Here's how the part is built. I have some questions about the finished solid (model axes, mm). A direction names the side the tool comes from. Round coordinates to 2 decimals unless told otherwise and drop trailing zeros. Write each loop counter-clockwise with the first axis right and the second up, starting at its lowest first coordinate (ties: lowest second). Pieces come first, ordered by that corner, then holes. Notation, with made-up numbers: M 62,15 L 80,15 A29 ccw 80,49 Z; hole C -16.75,-24.5 d11. An arc over 180 degrees is marked long. Write item = value, one per line. Start each with the question number.
(1) I need wall thicknesses on line 1 along Y through (x, z) = (35.5, 18.75); line 2 along Y through (x, z) = (-15.5, 4); line 3 along X through (y, z) = (-6.5, 10.5). Which ranges of each line are inside material? Lowest first, please.
(2) On a 3-axis mill with a long thin cutter (end or side, diameter ignored), from which of +Z, -Z, +X, -X, +Y, -Y can I reach the whole of each face in a straight line? I mean faces 5 (the flat face through (-0.367, 23.785, 22.535)), 6 (the flat face through (80, -35, 6)). Say none if no direction works.
(3) Will these pins go through, and if not, where does the flat tip stop? pin 1 Ø7.5 at (y, z) = (-9, 15.5) entering from -X; pin 2 Ø7.5 at (y, z) = (13.5, 10) entering from +X; pin 3 Ø2 at (x, z) = (64, 6) entering from +Y.
(4) I want a section at A-A (z = 3.5). Give the number of separate pieces and of enclosed holes in the cut face, and give its area (3 significant figures).
(5) I want a section at B-B (x = -15.5). List the corners of the cut face in (y, z) for me, and give its area (3 significant figures).
(6) If we mould it in two halves opening along X, with no side actions, what happens to faces 1 (the flat face through (-21.25, 0, 15)), 2 (the flat face through (65, -30, 12)), 3 (the cylindrical face through (51, -28, 13)), 4 (the cylindrical face through (13.9, 15.57, 4.93))? For each: released by +X, released by -X, zero draft, split by the parting line, or undercut.
(7) I want a section at D-D (y = 0). List the corners of the cut face in (x, z) for me.
(8) I want a section at C-C (y = -15.5). List the corners of the cut face in (x, z) for me.
```python
from build123d import *

# Parameters (mm, degrees)
F0_R      = 4.1
F0_W      = 42.5
F0_H      = 42.5
F0_W_2    = 30
F0_H_2    = 10
F1_DEPTH  = 25
F0_R_2    = 1.6
F0_R_3    = 6
F2_DEPTH  = 10
F3_SIZE   = 5
F4_R      = 5
F5_R      = 5
F6_R      = 2.1
F7_DEPTH  = 25
F8_R      = 12.5
F9_R      = 2.1
F10_DEPTH = 25


with BuildPart() as f1:
    # F0 (on Top) → F1 (new body)
    with BuildSketch(Plane.XY):
        Polygon((-50, -30), (-50, -40), (50, -40), (50, -30), (50, 40), (-50, 40), align=None)
        with Locations((-35.5, -30.5)):
            Circle(F0_R, mode=Mode.SUBTRACT)
        with Locations((35.5, -30.5)):
            Circle(F0_R, mode=Mode.SUBTRACT)
        with Locations((-35.5, 30.5)):
            Circle(F0_R, mode=Mode.SUBTRACT)
        Rectangle(F0_W, F0_H, mode=Mode.SUBTRACT)
        with Locations((35.5, 30.5)):
            Circle(F0_R, mode=Mode.SUBTRACT)
        with Locations((-65, -35)):
            Rectangle(F0_W_2, F0_H_2)
        with Locations((65, -35)):
            Rectangle(F0_W_2, F0_H_2)
    extrude(amount=F1_DEPTH)

    # F0 (on Top) → F2 (join)
    with BuildSketch(Plane.XY):
        Rectangle(F0_W, F0_H)
        with Locations((-15.5, -15.5)):
            Circle(F0_R_2, mode=Mode.SUBTRACT)
        with Locations((15.5, -15.5)):
            Circle(F0_R_2, mode=Mode.SUBTRACT)
        with Locations((-15.5, 15.5)):
            Circle(F0_R_2, mode=Mode.SUBTRACT)
        Circle(F0_R_3, mode=Mode.SUBTRACT)
        with Locations((15.5, 15.5)):
            Circle(F0_R_2, mode=Mode.SUBTRACT)
    extrude(amount=F2_DEPTH)

    # F3
    f3_edges = [f1.edges().sort_by_distance(p)[0] for p in [
        (-21.25, 0, 25),
        (0, 21.25, 25),
        (21.25, 0, 25),
        (0, -21.25, 25),
    ]]
    chamfer(f3_edges, length=F3_SIZE)

    # F4
    f4_edges = [f1.edges().sort_by_distance(p)[0] for p in [
        (-6, 0, 10),
    ]]
    fillet(f4_edges, radius=F4_R)

    # F5
    f5_edges = [f1.edges().sort_by_distance(p)[0] for p in [
        (50, -30, 12.5),
        (-50, -30, 12.5),
        (-50, 40, 12.5),
        (50, 40, 12.5),
    ]]
    fillet(f5_edges, radius=F5_R)

    # F6 (on face) → F7 (cut)
    with BuildSketch(Plane(origin=(0, -30, 0), x_dir=(-1, 0, 0), z_dir=(0, 1, 0))):
        with Locations((67.5, 12.5)):
            Circle(F6_R)
    extrude(amount=-F7_DEPTH, mode=Mode.SUBTRACT)

    # F8
    f8_edges = [f1.edges().sort_by_distance(p)[0] for p in [
        (-80, -35, 25),
        (80, -35, 25),
    ]]
    fillet(f8_edges, radius=F8_R)

    # F9 (on face) → F10 (cut)
    with BuildSketch(Plane(origin=(0, -30, 0), x_dir=(-1, 0, 0), z_dir=(0, 1, 0))):
        with Locations((-67.5, 12.5)):
            Circle(F9_R)
    extrude(amount=-F10_DEPTH, mode=Mode.SUBTRACT)


solid = f1.part
```
Returned:
q1.line_1 = -40 to -34.6, -26.4 to 26.4, 34.6 to 40
q1.line_2 = -40 to -17.1, -13.9 to 13.9, 17.1 to 40
q1.line_3 = -50 to -21.25, 21.25 to 50
q2.face_5 = +Z
q2.face_6 = +Z, -Z, +X, +Y, -Y
q3.pin_1 = -50
q3.pin_2 = 50
q3.pin_3 = -30
q4.separate_pieces = 1
q4.enclosed_holes = 9
q4.area = 8,240 mm²
q5.outline = M -40,0 L -17.1,0 L -17.1,10 L -21.25,10 L -21.25,20 L -26.25,25 L -40,25 Z; M -13.9,0 L 13.9,0 L 13.9,10 L -13.9,10 Z; M 17.1,0 L 40,0 L 40,25 L 26.25,25 L 21.25,20 L 21.25,10 L 17.1,10 Z
q5.area = 1,270 mm²
q6.face_1 = undercut
q6.face_2 = zero draft
q6.face_3 = released by +X
q6.face_4 = undercut
q7.outline = M -50,0 L -6,0 L -6,5 A5 ccw -11,10 L -21.25,10 L -21.25,20 L -26.25,25 L -50,25 Z; M 6,0 L 50,0 L 50,25 L 26.25,25 L 21.25,20 L 21.25,10 L 11,10 A5 ccw 6,5 Z
q8.outline = M -50,0 L -17.1,0 L -17.1,10 L -21.25,10 L -21.25,20 L -26.25,25 L -50,25 Z; M -13.9,0 L 13.9,0 L 13.9,10 L -13.9,10 Z; M 17.1,0 L 50,0 L 50,25 L 26.25,25 L 21.25,20 L 21.25,10 L 17.1,10 Z
